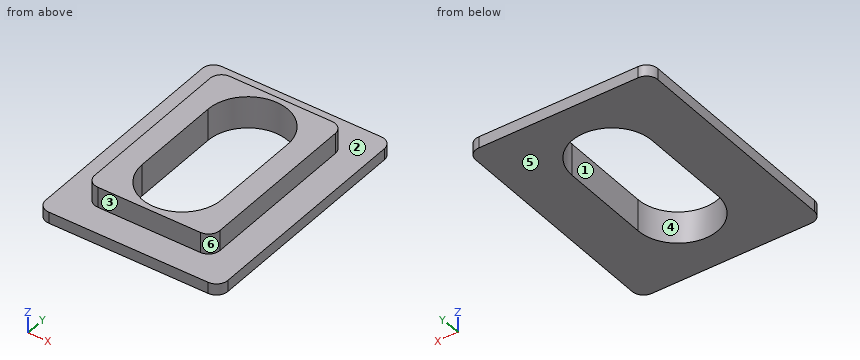
from build123d import *

# Parameters (mm, degrees)
RESSALTO_EXTRUS_O1_DEPTH = 1
RESSALTO_EXTRUS_O3_DEPTH = 2.8


with BuildPart() as part:
    # Esbo_o1 → Ressalto-extrus_o1 (new body)
    # profile 1 of 2: a face of its own
    with BuildSketch(Plane.XY):
        with BuildLine():
            ThreePointArc((1, 0), (0.292893219, 0.292893219), (0, 1))
            Line((0, 1), (0, 20))
            ThreePointArc((0, 20), (0.292893219, 20.707106781), (1, 21))
            Line((1, 21), (15, 21))
            ThreePointArc((15, 21), (15.707106781, 20.707106781), (16, 20))
            Line((16, 20), (16, 1))
            ThreePointArc((16, 1), (15.707106781, 0.292893219), (15, 0))
            Line((15, 0), (1, 0))
        make_face()
        with BuildLine():
            Line((3.5, 2.5), (12.5, 2.5))
            ThreePointArc((12.5, 2.5), (13.207106781, 2.792893219), (13.5, 3.5))
            Line((13.5, 3.5), (13.5, 17.5))
            ThreePointArc((13.5, 17.5), (13.207106781, 18.207106781), (12.5, 18.5))
            Line((12.5, 18.5), (3.5, 18.5))
            ThreePointArc((3.5, 18.5), (2.792893219, 18.207106781), (2.5, 17.5))
            Line((2.5, 17.5), (2.5, 3.5))
            ThreePointArc((2.5, 3.5), (2.792893219, 2.792893219), (3.5, 2.5))
        make_face(mode=Mode.SUBTRACT)
    # profile 2 of 2: a face of its own
    with BuildSketch(Plane.XY):
        with BuildLine():
            ThreePointArc((3.5, 2.5), (2.792893219, 2.792893219), (2.5, 3.5))
            Line((2.5, 3.5), (2.5, 17.5))
            ThreePointArc((2.5, 17.5), (2.792893219, 18.207106781), (3.5, 18.5))
            Line((3.5, 18.5), (12.5, 18.5))
            ThreePointArc((12.5, 18.5), (13.207106781, 18.207106781), (13.5, 17.5))
            Line((13.5, 17.5), (13.5, 3.5))
            ThreePointArc((13.5, 3.5), (13.207106781, 2.792893219), (12.5, 2.5))
            Line((12.5, 2.5), (3.5, 2.5))
        make_face()
        with BuildLine():
            ThreePointArc((11.5, 14.5), (8, 18), (4.5, 14.5))
            Line((4.5, 14.5), (4.5, 6.5))
            ThreePointArc((4.5, 6.5), (8, 3), (11.5, 6.5))
            Line((11.5, 6.5), (11.5, 14.5))
        make_face(mode=Mode.SUBTRACT)
    extrude(amount=RESSALTO_EXTRUS_O1_DEPTH)

    # Esbo_o1_4 → Ressalto-extrus_o3 (add)
    with BuildSketch(Plane.XY):
        with BuildLine():
            ThreePointArc((3.5, 2.5), (2.792893219, 2.792893219), (2.5, 3.5))
            Line((2.5, 3.5), (2.5, 17.5))
            ThreePointArc((2.5, 17.5), (2.792893219, 18.207106781), (3.5, 18.5))
            Line((3.5, 18.5), (12.5, 18.5))
            ThreePointArc((12.5, 18.5), (13.207106781, 18.207106781), (13.5, 17.5))
            Line((13.5, 17.5), (13.5, 3.5))
            ThreePointArc((13.5, 3.5), (13.207106781, 2.792893219), (12.5, 2.5))
            Line((12.5, 2.5), (3.5, 2.5))
        make_face()
        with BuildLine():
            ThreePointArc((11.5, 14.5), (8, 18), (4.5, 14.5))
            Line((4.5, 14.5), (4.5, 6.5))
            ThreePointArc((4.5, 6.5), (8, 3), (11.5, 6.5))
            Line((11.5, 6.5), (11.5, 14.5))
        make_face(mode=Mode.SUBTRACT)
    extrude(amount=RESSALTO_EXTRUS_O3_DEPTH)


solid = part.part
Geometry check sheet. Reference: the model listing, model coordinates, mm. Face numbers are marked on the shaded views. A direction names the side the tool comes from. Coordinates: 2 decimals unless noted, no trailing zeros. Order: outer loops, then holes, each group sorted by start corner. A loop starts at its lowest first (then second) coordinate and runs counter-clockwise, first axis right, second up. Notation, with made-up numbers: (-19.75, -23) -> (-10.75, -23) arc R15 cw to (-10.75, 5) -> close; hole circle Ø1 at (52, -33.75). An arc over 180 degrees is marked (long way). Use a Markdown table: item, result. Add a question column.
1. Cross-section at C-C (z = 1.75). Enter the section's corners in (x, y), and give its area (3 significant figures).
2. Material ranges on L1, parallel to X at y = 10.5, z = 1.8; L2, parallel to Y at x = 8.25, z = 1.55; L3, parallel to Y at x = 11.75, z = 1.75, recorded low to high.
3. Cross-section at A-A (x = 8). Enter the section's corners in (y, z).
4. Set-up check for the marked faces 1, 2 and 3: record each of +Z, -Z, +X, -X, +Y, -Y from which the full face is reachable in a straight line by a thin tool's end or side.
5. Go/stop test with flat-tipped pins: pin 1 Ø0.5 at (y, z) = (10.5, 2) entering from +X; pin 2 Ø0.5 at (x, z) = (8, 1.5) entering from -Y; pin 3 Ø0.9 at (x, z) = (9, 1.5) entering from +Y. Record where each tip stops, or that it passes through.
6. Cross-section at B-B (y = 7). Enter the section's corners in (x, z).
7. Mould release check, pull along X, two halves, no side actions. Record for the marked faces 4, 5 and 6: pulls with the +X half, pulls with the -X half, needs draft (parallel to the pull), parting line crosses it, or undercut.
8. Cross-section at D-D (x = 13.25). Enter the section's corners in (y, z), and give its area (3 significant figures).
Filled sheet:
| question | item | result |
|---|---|---|
| 1 | outline | (2.5, 3.5) arc R1 ccw to (3.5, 2.5) -> (12.5, 2.5) arc R1 ccw to (13.5, 3.5) -> (13.5, 17.5) arc R1 ccw to (12.5, 18.5) -> (3.5, 18.5) arc R1 ccw to (2.5, 17.5) -> close; hole (4.5, 6.5) arc R3.5 ccw to (11.5, 6.5) -> (11.5, 14.5) arc R3.5 ccw to (4.5, 14.5) -> close |
| 1 | area | 80.7 mm2 |
| 2 | L1 | 2.5 to 4.5, 11.5 to 13.5 |
| 2 | L2 | 2.5 to 3.01, 17.99 to 18.5 |
| 2 | L3 | 2.5 to 18.5 |
| 3 | outline | (0, 0) -> (3, 0) -> (3, 2.8) -> (2.5, 2.8) -> (2.5, 1) -> (0, 1) -> close; (18, 0) -> (21, 0) -> (21, 1) -> (18.5, 1) -> (18.5, 2.8) -> (18, 2.8) -> close |
| 4 | face 1 | +Z, -Z |
| 4 | face 2 | +Z |
| 4 | face 3 | +Z, +X, -X, -Y |
| 5 | pin 1 | x = 13.5 |
| 5 | pin 2 | y = 2.5 |
| 5 | pin 3 | y = 18.5 |
| 6 | outline | (0, 0) -> (4.5, 0) -> (4.5, 2.8) -> (2.5, 2.8) -> (2.5, 1) -> (0, 1) -> close; (11.5, 0) -> (16, 0) -> (16, 1) -> (13.5, 1) -> (13.5, 2.8) -> (11.5, 2.8) -> close |
| 7 | face 4 | undercut |
| 7 | face 5 | needs draft |
| 7 | face 6 | pulls with the +X half |
| 8 | outline | (0, 0) -> (21, 0) -> (21, 1) -> (18.16, 1) -> (18.16, 2.8) -> (2.84, 2.8) -> (2.84, 1) -> (0, 1) -> close |
| 8 | area | 48.6 mm2 |
